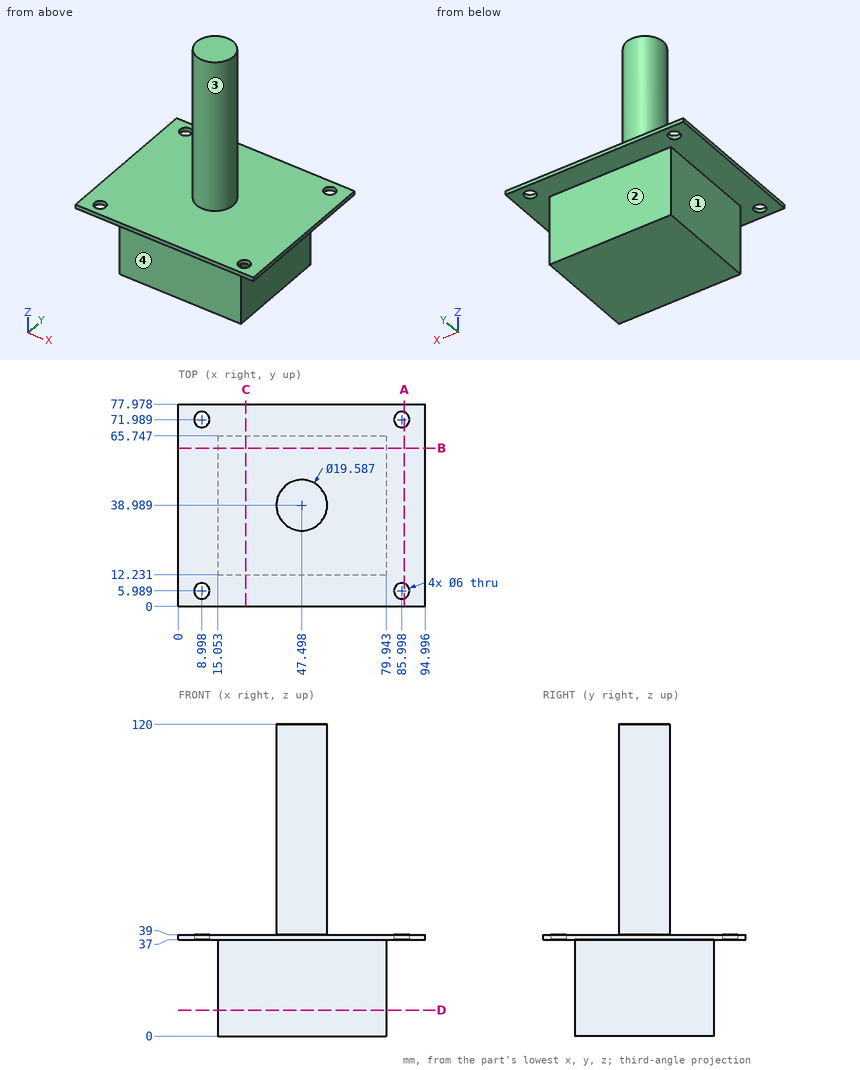
Source: three-view drawing plus pictorial views. Frame: mm from the lowest corner of the part. A direction names the side the tool comes from. Give positions to 0.01 mm unless a question says otherwise; leave off trailing zeros. Order: outer loops, then holes, each group sorted by start corner. A loop starts at its lowest first (then second) coordinate and runs counter-clockwise, first axis right, second up. Notation, with made-up numbers: M -15.75,-35.5 L 8.25,-35.5 A24 ccw 8.25,-18.5 Z; hole C 14.25,-21.5 d2. An arc over 180 degrees is marked long. Return JSON: item names as keys, results as strings.
Item 1: Cut plane B-B (y = 61). Return loops of the section in (x, z), then the cut area to 3 significant figures.
Solutions:
{"outline": "M 0,37 L 15.05,37 L 15.05,0 L 79.94,0 L 79.94,37 L 95,37 L 95,39 L 0,39 Z", "area": "2,590 mm^2"}
Item 2: Access query for the marked faces 1, 2, 3 and 4. Directions: +Z, -Z, +X, -X, +Y, -Y. A direction counts if a zero-diameter tool reaches every point of the face in a straight line with its end or side. Return the directions, or none.
Solutions:
{"face 1": "-Z, -X, +Y, -Y", "face 2": "-Z, +X, -X, +Y", "face 3": "+Z", "face 4": "-Z, +X, -X, -Y"}
Item 3: Cut plane D-D (z = 10). Return loops of the section in (x, y).
Solutions:
{"outline": "M 15.05,12.23 L 79.94,12.23 L 79.94,65.75 L 15.05,65.75 Z"}
Item 4: Ray query, probe 1 along Z at (x, y) = (35, 36); probe 2 along Y at (x, z) = (48, 102); probe 3 along Z at (x, y) = (9.5, 36). Return the intervals inside material, ascending.
Solutions:
{"probe 1": "0 to 39", "probe 2": "29.21 to 48.77", "probe 3": "37 to 39"}
Item 5: Cut plane C-C (x = 26). Return loops of the section in (y, z), then the cut area to 3 significant figures.
Solutions:
{"outline": "M 0,37 L 12.23,37 L 12.23,0 L 65.75,0 L 65.75,37 L 77.98,37 L 77.98,39 L 0,39 Z", "area": "2,140 mm^2"}
Item 6: Cut plane A-A (x = 87). Return loops of the section in (y, z), then the cut area to 3 significant figures.
Solutions:
{"outline": "M 0,37 L 3.16,37 L 3.16,39 L 0,39 Z; M 8.82,37 L 69.16,37 L 69.16,39 L 8.82,39 Z; M 74.82,37 L 77.98,37 L 77.98,39 L 74.82,39 Z", "area": "133 mm^2"}
Item 7: First-contact query: P1, Ø2, axis at y = 29.5, z = 59, coming from the +X side; P2, Ø11, axis at x = 52, z = 11.5, coming from the -Y side; P3, Ø11, axis at y = 30.5, z = 14, coming from the +X side; P4, Ø5, axis at y = 37.5, z = 36.5, coming from the +X side. Flat tips, straight axial feed; report the tip coordinate or a pass-through.
Solutions:
{"P1": "x = 52.38", "P2": "y = 12.23", "P3": "x = 79.94", "P4": "x = 95"}
